```python
from build123d import *

# Parameters (mm, degrees)
FILLET1_R                 = 2.54
CHAMFER1_SIZE             = 2.54
F_8_32_TAPPED_HOLE1_D     = 3.4544
F_8_32_TAPPED_HOLE1_DEPTH = 10.668
F_8_32_TAPPED_HOLE1_TIP   = 1.037806461


with BuildPart() as part:
    # Sketch1 → Revolve1 (revolve)
    with BuildSketch(Plane.XY):
        Polygon((-8.89, 26.005455731), (-8.89, 19.655455731), (-38.219393675, -31.144544269), (-39.37, -31.144544269), (-39.37, 19.655455731), (-11.43, 19.655455731), (-11.43, 26.005455731), align=None)
    revolve(axis=Axis((0, 33.494633817, 0), (0, -1, 0)))

    # Fillet1
    fillet1_edges = [part.edges().sort_by_distance(p)[0] for p in [
        (11.43, 19.655455731, 0),
    ]]
    fillet(fillet1_edges, radius=FILLET1_R)

    # Chamfer1
    chamfer1_edges = [part.edges().sort_by_distance(p)[0] for p in [
        (39.37, 19.655455731, 0),
    ]]
    chamfer(chamfer1_edges, length=CHAMFER1_SIZE)

    # #8-32 Tapped Hole1
    with Locations(Plane(origin=(0, 19.655455731, 0), x_dir=(1, 0, 0), z_dir=(0, 1, 0))):
        with Locations((0, -25.4), (25.4, 0), (0, 25.4), (-25.4, 0)):
            Hole(F_8_32_TAPPED_HOLE1_D / 2, depth=F_8_32_TAPPED_HOLE1_DEPTH)
            with Locations((0, 0, -(F_8_32_TAPPED_HOLE1_DEPTH + F_8_32_TAPPED_HOLE1_TIP / 2))):  # 118° drill point
                Cone(0, F_8_32_TAPPED_HOLE1_D / 2, F_8_32_TAPPED_HOLE1_TIP, mode=Mode.SUBTRACT)


solid = part.part
```
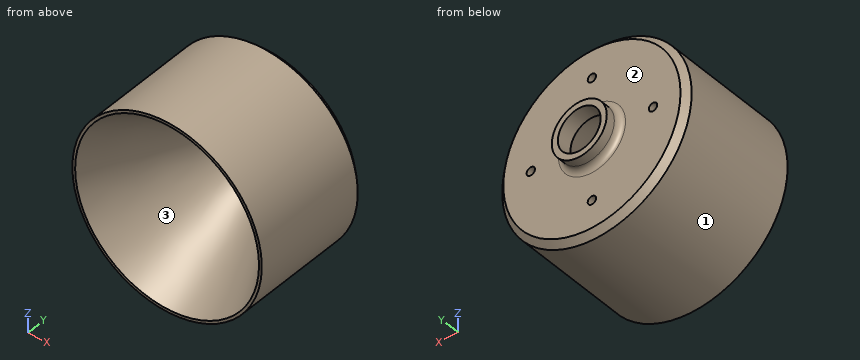
Can you work these out from the model? Positions are in its coordinate system, mm. Face numbers are marked on the shaded views. Round coordinates to 2 decimals unless told otherwise and drop trailing zeros.
Item 1: If we mould it in two halves opening along Z, with no side actions, what happens to the marked faces 1, 2 and 3? For each: +Z half, -Z half, draft (parallel to the pull), parting line (faces both ways), or undercut.
Item 2: Will these pins go through, and if not, where does the flat tip stop? pin 1 Ø12 at (x, y) = (24, 4.5) entering from +Z; pin 2 Ø2 at (y, z) = (12.5, 14) entering from -X; pin 3 Ø5.5 at (x, z) = (0, -25.4) entering from -Y.
Item 3: Please list where these lines run through material, in increasing order: L1, parallel to Z at x = -24.5, y = -26; L2, parallel to X at y = -21, z = 21; L3, parallel to X at y = 10, z = -24.
Reported:
1. face 1: parting line
1. face 2: draft
1. face 3: undercut
2. pin 1: stops at z = 35.01
2. pin 2: stops at x = -37.16
2. pin 3: stops at y = -13.7
3. L1: z = -30.82 to -25.34, 25.34 to 30.82
3. L2: x = -33.3 to -24.62, 24.62 to 33.3
3. L3: x = -31.21 to -1.01, 1.01 to 31.21
